```python
from build123d import *

# Parameters (mm, degrees)
SKETCH1_W            = 27
SKETCH1_H            = 18
BOSS_EXTRUDE1_DEPTH  = 26
SKETCH2_W            = 12.5
SKETCH2_H            = 12.5
CUT_EXTRUDE1_DEPTH   = 26
SKETCH4_W            = 26
SKETCH4_H            = 18
BOSS_EXTRUDE2_DEPTH  = 5
SKETCH5_W            = 12.5
SKETCH5_H            = 12.5
CUT_EXTRUDE2_DEPTH   = 26
SKETCH7_W            = 26
SKETCH7_H            = 1
BOSS_EXTRUDE3_DEPTH  = 8
SKETCH8_W            = 48
SKETCH8_H            = 8
BOSS_EXTRUDE4_DEPTH  = 1
SKETCH9_W            = 5
SKETCH9_H            = 4
CUT_EXTRUDE4_DEPTH   = 8
SKETCH10_W           = 48
SKETCH10_H           = 32
BOSS_EXTRUDE5_DEPTH  = 1
SKETCH12_W           = 5
SKETCH12_H           = 3
BOSS_EXTRUDE7_DEPTH  = 10
SKETCH14_W           = 3
SKETCH14_H           = 5
SKETCH14_H_2         = 4
BOSS_EXTRUDE8_DEPTH  = 10
BOSS_EXTRUDE9_DEPTH  = 1
SKETCH17_W           = 38
SKETCH17_H           = 2.75142147
BOSS_EXTRUDE11_DEPTH = 10
BOSS_EXTRUDE12_DEPTH = 10
BOSS_EXTRUDE13_DEPTH = 22
SKETCH21_W           = 32
SKETCH21_H           = 18
CUT_EXTRUDE5_DEPTH   = 1
SKETCH22_W           = 22
SKETCH22_H           = 18
BOSS_EXTRUDE14_DEPTH = 8
CUT_EXTRUDE6_DEPTH   = 40
BOSS_EXTRUDE17_DEPTH = 10


with BuildPart() as part:
    # Sketch1 → Boss-Extrude1 (new body)
    with BuildSketch(Plane(origin=(0, 0, 0), x_dir=(0, 0, -1), z_dir=(1, 0, 0))):
        with Locations((13.5, 9)):
            Rectangle(SKETCH1_W, SKETCH1_H)
    extrude(amount=BOSS_EXTRUDE1_DEPTH)

    # Sketch2 → Cut-Extrude1 (cut)
    with BuildSketch(Plane(origin=(26, 0, 0), x_dir=(0, 0, -1), z_dir=(1, 0, 0))):
        with Locations((9.25, 8.25)):
            Rectangle(SKETCH2_W, SKETCH2_H)
    extrude(amount=-CUT_EXTRUDE1_DEPTH, mode=Mode.SUBTRACT)

    # Sketch4 → Boss-Extrude2 (add)
    with BuildSketch(Plane(origin=(0, 0, -27), x_dir=(-1, 0, 0), z_dir=(0, 0, -1))):
        with Locations((-13, 9)):
            Rectangle(SKETCH4_W, SKETCH4_H)
    extrude(amount=BOSS_EXTRUDE2_DEPTH)

    # Sketch5 → Cut-Extrude2 (cut)
    with BuildSketch(Plane(origin=(26, 0, 0), x_dir=(0, 0, -1), z_dir=(1, 0, 0))):
        with Locations((22.75, 8.25)):
            Rectangle(SKETCH5_W, SKETCH5_H)
    extrude(amount=-CUT_EXTRUDE2_DEPTH, mode=Mode.SUBTRACT)

    # Sketch7 → Boss-Extrude3 (add)
    with BuildSketch(Plane.XY):
        with Locations((13, 0.5)):
            Rectangle(SKETCH7_W, SKETCH7_H)
    extrude(amount=BOSS_EXTRUDE3_DEPTH)

    # Sketch8 → Boss-Extrude4 (add)
    with BuildSketch(Plane(origin=(0, 1, 0), x_dir=(1, 0, 0), z_dir=(0, 1, 0))):
        with Locations((13, -4)):
            Rectangle(SKETCH8_W, SKETCH8_H)
    extrude(amount=-BOSS_EXTRUDE4_DEPTH)

    # Sketch9 → Cut-Extrude4 (cut)
    with BuildSketch(Plane(origin=(0, 1, 0), x_dir=(1, 0, 0), z_dir=(0, 1, 0))):
        with Locations((-8.5, -4)):
            Rectangle(SKETCH9_W, SKETCH9_H)
        with Locations((34.5, -4)):
            Rectangle(SKETCH9_W, SKETCH9_H)
    extrude(amount=-CUT_EXTRUDE4_DEPTH, mode=Mode.SUBTRACT)

    # Sketch10 → Boss-Extrude5 (add)
    with BuildSketch(Plane(origin=(0, 18, 0), x_dir=(1, 0, 0), z_dir=(0, 1, 0))):
        with Locations((13, 16)):
            Rectangle(SKETCH10_W, SKETCH10_H)
    extrude(amount=BOSS_EXTRUDE5_DEPTH)

    # Sketch12 → Boss-Extrude7 (add)
    with BuildSketch(Plane(origin=(0, 19, 0), x_dir=(1, 0, 0), z_dir=(0, 1, 0))):
        with Locations((-8.5, 14.5)):
            Rectangle(SKETCH12_W, SKETCH12_H)
        with Locations((34.5, 14.5)):
            Rectangle(SKETCH12_W, SKETCH12_H)
    extrude(amount=BOSS_EXTRUDE7_DEPTH)

    # Sketch14 → Boss-Extrude8 (add)
    with BuildSketch(Plane(origin=(0, 19, 0), x_dir=(1, 0, 0), z_dir=(0, 1, 0))):
        with Locations((3.5, 2.5)):
            Rectangle(SKETCH14_W, SKETCH14_H)
        with Locations((22.5, 2)):
            Rectangle(SKETCH14_W, SKETCH14_H_2)
    extrude(amount=BOSS_EXTRUDE8_DEPTH)

    # Sketch15 → Boss-Extrude9 (add)
    with BuildSketch(Plane(origin=(0, 29, 0), x_dir=(1, 0, 0), z_dir=(0, 1, 0))):
        Polygon((2, 0), (-11, 13), (-11, 16), (-11, 32), (37, 32), (37, 13), (24, 0), align=None)
    extrude(amount=BOSS_EXTRUDE9_DEPTH)

    # Sketch17 → Boss-Extrude11 (add)
    with BuildSketch(Plane(origin=(0, 30, 0), x_dir=(1, 0, 0), z_dir=(0, 1, 0))):
        with Locations((13, 30.624289265)):
            Rectangle(SKETCH17_W, SKETCH17_H)
    extrude(amount=BOSS_EXTRUDE11_DEPTH)



with BuildPart() as body_2:
    # Sketch18 → Boss-Extrude12 (new body)
    with BuildSketch(Plane(origin=(0, 30, 0), x_dir=(1, 0, 0), z_dir=(0, 1, 0))):
        Polygon((2, 0), (4.75142147, -2.75142147), (21.24857853, -2.75142147), (24, 0), align=None)
    extrude(amount=BOSS_EXTRUDE12_DEPTH)


with BuildPart() as part_1:
    add(part.part)

    add(body_2.part)  # Boss-Extrude13 merges body 2
    # Sketch19 → Boss-Extrude13 (add)
    with BuildSketch(Plane(origin=(2, 30, 0), x_dir=(0, 0, 1), z_dir=(-1, 0, 0))):
        Polygon((0, -1), (2.75142147, 0), (0, 0), align=None)
    extrude(amount=-BOSS_EXTRUDE13_DEPTH)

    # Sketch21 → Cut-Extrude5 (cut)
    with BuildSketch(Plane(origin=(0, 30, 0), x_dir=(1, 0, 0), z_dir=(0, 1, 0))):
        with Locations((13, 23)):
            Rectangle(SKETCH21_W, SKETCH21_H)
    extrude(amount=-CUT_EXTRUDE5_DEPTH, mode=Mode.SUBTRACT)

    # Sketch22 → Boss-Extrude14 (add)
    with BuildSketch(Plane.XY):
        with Locations((13, 10)):
            Rectangle(SKETCH22_W, SKETCH22_H)
    extrude(amount=BOSS_EXTRUDE14_DEPTH)

    # Sketch23 → Cut-Extrude6 (cut)
    with BuildSketch(Plane(origin=(24, 0, 0), x_dir=(0, 0, -1), z_dir=(1, 0, 0))):
        Polygon((0, 19), (-4, 3), (-8, 1), (-8, 19), align=None)
    extrude(amount=-CUT_EXTRUDE6_DEPTH, mode=Mode.SUBTRACT)

    # Sketch25 → Boss-Extrude17 (add)
    with BuildSketch(Plane(origin=(0, 30, 0), x_dir=(1, 0, 0), z_dir=(0, 1, 0))):
        Polygon((24, 0), (37, 13), (37, 22.5), (22, 0), align=None)
        Polygon((2, 0), (-11, 13), (-11, 22.5), (4, 0), align=None)
    extrude(amount=BOSS_EXTRUDE17_DEPTH)


solid = part_1.part
```
Design review of the part built by this model. Coordinates are the model's own, in mm. A direction names the side the tool comes from. Round coordinates to 2 decimals unless told otherwise and drop trailing zeros. Write each loop counter-clockwise with the first axis right and the second up, starting at its lowest first coordinate (ties: lowest second). Pieces come first, ordered by that corner, then holes. Notation, with made-up numbers: (78, 16) -> (102, 16) arc R16 cw to (102, 40) -> close; hole circle Ø11 at (22, 74). An arc over 180 degrees is marked (long way). Write item = value, one per line. Start each with the question number.
1) Wall thickness on probe 1 along Y at (x, z) = (27, -29.5); probe 2 along Y at (x, z) = (32.5, -28); probe 3 along Z at (x, y) = (13, 11): over which ranges is each line inside the solid? List them lowest first. Write a range as from..to.
2) Tool access review of faces 4 (the face through (3, 30, 2)), 5 (the face through (13, 35, -29.249)), 6 (the face through (32, 35, -31)), 7 (the face through (21, 24, -2)): name each direction out of +Z, -Z, +X, -X, +Y, -Y from which nothing blocks a thin tool from reaching the whole face with its end or side.
3) Mouldability with a two-part tool opening along Y and no side actions: class faces 1 (the face through (13, 40, -31)), 2 (the face through (29.6, 34.9, -11.4)), 3 (the face through (13, 2, -9)) as +Y half, -Y half, draft (parallel to the pull), parting line (faces both ways), or undercut.
4) Take a section at A-A, the plane x = 10. State the section outline as (y, z) points.
5) Take a section at D-D, the plane y = 33. State the section outline as (x, z) points.
6) Take a section at C-C, the plane y = 9. State the section outline as (x, z) points, plus the area to 3 significant figures.
7) Take a section at B-B, the plane x = 23. State the section outline as (y, z) points, plus the area to 3 significant figures.
8) Clearance check with flat-ended pins moving along their axes: pin 1 (10 mm diameter, centred on y = 10.5, z = -2, fed in from +X); pin 2 (10 mm diameter, centred on x = -6, z = -22, fed in from -Y); pin 3 (4 mm diameter, centred on x = 8, y = 9.5, fed in from +Z) (3 decimals); pin 4 (4 mm diameter, centred on y = 6.5, z = 5.5, fed in from +X). State where each tip first meets the part, or that it passes through.
Results list:
q1.probe_1 = 18..19, 30..40
q1.probe_2 = 18..19, 29..30
q1.probe_3 = -32..-29, -16.5..-15.5, -3..2
q2.face_4 = +Z, -X, +Y
q2.face_5 = +X, -X, +Y
q2.face_6 = -Z, +X, +Y
q2.face_7 = +Z, -Z
q3.face_1 = +Y half
q3.face_2 = draft
q3.face_3 = undercut
q4.outline = (0, -32) -> (19, -32) -> (19, 0) -> (3, 4) -> (1, 8) -> (0, 8) -> close; (29, -14) -> (30, -14) -> (30, 0) -> (40, 0) -> (40, 2.75) -> (30, 2.75) -> (29, 0) -> close; (30, -32) -> (40, -32) -> (40, -29.25) -> (30, -29.25) -> close; hole (2, -29) -> (14.5, -29) -> (14.5, -16.5) -> (2, -16.5) -> close; hole (2, -15.5) -> (14.5, -15.5) -> (14.5, -3) -> (2, -3) -> close
q5.outline = (-11, -22.5) -> (4, 0) -> (22, 0) -> (37, -22.5) -> (37, -13) -> (21.25, 2.75) -> (4.75, 2.75) -> (-11, -13) -> close; (-6, -32) -> (32, -32) -> (32, -29.25) -> (-6, -29.25) -> close
q6.outline = (0, -32) -> (26, -32) -> (26, -29) -> (0, -29) -> close; (0, -16.5) -> (26, -16.5) -> (26, -15.5) -> (0, -15.5) -> close; (0, -3) -> (26, -3) -> (26, 0) -> (24, 0) -> (24, 2.5) -> (2, 2.5) -> (2, 0) -> (0, 0) -> close
q6.area = 237 mm²
q7.outline = (0, -32) -> (19, -32) -> (19, -4) -> (29, -4) -> (29, -14) -> (30, -14) -> (30, -1.5) -> (40, -1.5) -> (40, 1) -> (30, 1) -> (30, 2.75) -> (29, 0) -> (19, 0) -> (3, 4) -> (1, 8) -> (0, 8) -> close; (30, -32) -> (40, -32) -> (40, -29.25) -> (30, -29.25) -> close; hole (2, -29) -> (14.5, -29) -> (14.5, -16.5) -> (2, -16.5) -> close; hole (2, -15.5) -> (14.5, -15.5) -> (14.5, -3) -> (2, -3) -> close
q7.area = 455 mm²
q8.pin_1 = 26
q8.pin_2 = 18
q8.pin_3 = 2.875
q8.pin_4 = through
